Input: part model. Units: mm. Frame: model coordinates. Face numbers are marked on the shaded views. A direction names the side the tool comes from. Coordinates: 2 decimals unless noted, no trailing zeros. Write each loop counter-clockwise with the first axis right and the second up, starting at its lowest first coordinate (ties: lowest second). Pieces come first, ordered by that corner, then holes. Notation, with made-up numbers: M 48.25,-13 L 91.25,-13 A8 cw 91.25,-7 Z; hole C 52,-38 d2. An arc over 180 degrees is marked long. Write each question's results on one line, items separated by ' | '. Start each with the question number.
1. Section query D-D, the plane z = 7.5. Output: boundary loops of the cut face in (x, y).
2. Section query A-A, the plane x = 15.5. Count the separate pieces of the cut face and the enclosed holes in it, and give its area (3 significant figures).
3. Ray query, probe 1 along Z at (x, y) = (-15.5, -6.1); probe 2 along Y at (x, z) = (14.5, 25.5); probe 3 along Z at (x, y) = (-20.5, -26). Return the intervals inside material, ascending.
4. Section query B-B, the plane y = -21. Output: boundary loops of the cut face in (x, z).
5. First-contact query: pin 1 (4 mm diameter, centred on x = -15.5, z = 15.36, fed in from -Y); pin 2 (1 mm diameter, centred on x = 3, y = -34.5, fed in from +Z). Flat tips, straight axial feed; report the tip coordinate or a pass-through.
6. Set-up query: the marked faces 1 and 2. Return all of +Z, -Z, +X, -X, +Y, -Y with unobstructed straight access to the full face (end or side cutting, diameter ignored); none if empty.
7. Pull-direction query (X, two-part tool) for the marked faces 3, 4 and 5; classes: +X half, -X half, draft (parallel to the pull), parting line (faces both ways), or undercut.
```python
from build123d import *

# Parameters (mm, degrees)
SCHIZZO1_R                             = 1.75
SCHIZZO1_R_2                           = 11.05
SCHIZZO1_R_3                           = 2
BASE_FLANGIA1_DEPTH                    = 4
PIEGATURA_START                        = -3.5
PIEGATURA_DELLO_SCHIZZO1_OUTLINE_W     = 50
PIEGATURA_DELLO_SCHIZZO1_OUTLINE_H     = 4
PIEGATURA_DELLO_SCHIZZO1_DEPTH         = 51
PIEGATURA_START_2                      = -7.5
PIEGATURA_DELLO_SCHIZZO1_2_OUTLINE_R   = 1.75
PIEGATURA_DELLO_SCHIZZO1_2_OUTLINE_R_2 = 11.05
PIEGATURA_DELLO_SCHIZZO1_2_DEPTH       = 4
PIEGATURA_START_3                      = -26
PIEGATURA_DELLO_SCHIZZO1_3_DEPTH       = 52
PIEGATURA_START_4                      = -25
PIEGATURA_DELLO_SCHIZZO1_4_DEPTH       = 50
ESTRUSIONE_ESTRUSIONE1_DEPTH           = 2


with BuildPart() as part:
    # Base-Flangia1: sheet metal written as solids
    # Schizzo1 → Base-Flangia1 (new body)
    with BuildSketch(Plane.XY):
        with BuildLine():
            Line((-25, 42.5), (-20, 47.5))
            Line((-20, 47.5), (20, 47.5))
            Line((20, 47.5), (25, 42.5))
            Line((25, 42.5), (25, -42.5))
            ThreePointArc((25, -42.5), (23.535533906, -46.035533906), (20, -47.5))
            Line((20, -47.5), (-20, -47.5))
            ThreePointArc((-20, -47.5), (-23.535533906, -46.035533906), (-25, -42.5))
            Line((-25, -42.5), (-25, 42.5))
        make_face()
        with Locations((-15.5, 42)):
            Circle(SCHIZZO1_R, mode=Mode.SUBTRACT)
        with Locations((15.5, 42)):
            Circle(SCHIZZO1_R, mode=Mode.SUBTRACT)
        with Locations((15.5, 11)):
            Circle(SCHIZZO1_R, mode=Mode.SUBTRACT)
        with Locations((-15.5, 11)):
            Circle(SCHIZZO1_R, mode=Mode.SUBTRACT)
        with Locations((0, 26.5)):
            Circle(SCHIZZO1_R_2, mode=Mode.SUBTRACT)
        with Locations((-12.5, -37.5)):
            Circle(SCHIZZO1_R_3, mode=Mode.SUBTRACT)
        with Locations((12.5, -37.5)):
            Circle(SCHIZZO1_R_3, mode=Mode.SUBTRACT)
    extrude(amount=-BASE_FLANGIA1_DEPTH)

    # Piegatura dello schizzo1: read off the stored shape, not the designer's step
    # Piegatura dello schizzo1 outline → Piegatura dello schizzo1 (cut)
    with BuildSketch(Plane(origin=(0, 0, 0), x_dir=(1, 0, 0), z_dir=(0, 1, 0)).offset(PIEGATURA_START)):
        with Locations((0, 2)):
            Rectangle(PIEGATURA_DELLO_SCHIZZO1_OUTLINE_W, PIEGATURA_DELLO_SCHIZZO1_OUTLINE_H)
    extrude(amount=PIEGATURA_DELLO_SCHIZZO1_DEPTH, mode=Mode.SUBTRACT)

    # Piegatura dello schizzo1 2 outline → Piegatura dello schizzo1 2 (add)
    with BuildSketch(Plane(origin=(0, 0, 0), x_dir=(1, 0, 0), z_dir=(0, 1, 0)).offset(PIEGATURA_START_2)):
        Polygon((-25, 0), (-25, -46.862699383), (-20, -51.862699383), (20, -51.862699383), (25, -46.862699383), (25, 0), align=None)
        with Locations((-15.5, -46.362699383)):
            Circle(PIEGATURA_DELLO_SCHIZZO1_2_OUTLINE_R, mode=Mode.SUBTRACT)
        with Locations((15.5, -46.362699383)):
            Circle(PIEGATURA_DELLO_SCHIZZO1_2_OUTLINE_R, mode=Mode.SUBTRACT)
        with Locations((0, -30.862699383)):
            Circle(PIEGATURA_DELLO_SCHIZZO1_2_OUTLINE_R_2, mode=Mode.SUBTRACT)
        with Locations((-15.5, -15.362699383)):
            Circle(PIEGATURA_DELLO_SCHIZZO1_2_OUTLINE_R, mode=Mode.SUBTRACT)
        with Locations((15.5, -15.362699383)):
            Circle(PIEGATURA_DELLO_SCHIZZO1_2_OUTLINE_R, mode=Mode.SUBTRACT)
    extrude(amount=PIEGATURA_DELLO_SCHIZZO1_2_DEPTH)

    # Piegatura dello schizzo1 3 outline → Piegatura dello schizzo1 3 (cut)
    with BuildSketch(Plane.YZ.offset(PIEGATURA_START_3)):
        with BuildLine():
            ThreePointArc((-3.5, 0.01), (-4.674501807, -2.825498193), (-7.51, -4))
            Line((-7.51, -4), (-3.5, -4))
            Line((-3.5, -4), (-3.5, 0.01))
        make_face()
    extrude(amount=PIEGATURA_DELLO_SCHIZZO1_3_DEPTH, mode=Mode.SUBTRACT)

    # Piegatura dello schizzo1 4 outline → Piegatura dello schizzo1 4 (add)
    with BuildSketch(Plane.YZ.offset(PIEGATURA_START_4)):
        with BuildLine():
            ThreePointArc((-7.5, 0.01), (-7.502928932, 0.002928932), (-7.51, 0))
            Line((-7.51, 0), (-7.5, 0))
            Line((-7.5, 0), (-7.5, 0.01))
        make_face()
    extrude(amount=PIEGATURA_DELLO_SCHIZZO1_4_DEPTH)

    # Schizzo13 → Estrusione-Estrusione1 (add)
    with BuildSketch(Plane.ZY.offset(25)):
        with BuildLine():
            Line((0.01, -7.5), (15, -7.5))
            Line((15, -7.5), (0, -22.5))
            Line((0, -22.5), (0, -7.51))
            ThreePointArc((0, -7.51), (0.002928932, -7.502928932), (0.01, -7.5))
        make_face()
    estrusione_estrusione1 = extrude(amount=-ESTRUSIONE_ESTRUSIONE1_DEPTH)

    # Specchia1: Estrusione-Estrusione1 across plane
    add(estrusione_estrusione1.mirror(Plane(origin=(0, 0, 0), x_dir=(0, 0, 1), z_dir=(1, 0, 0))))


solid = part.part
```
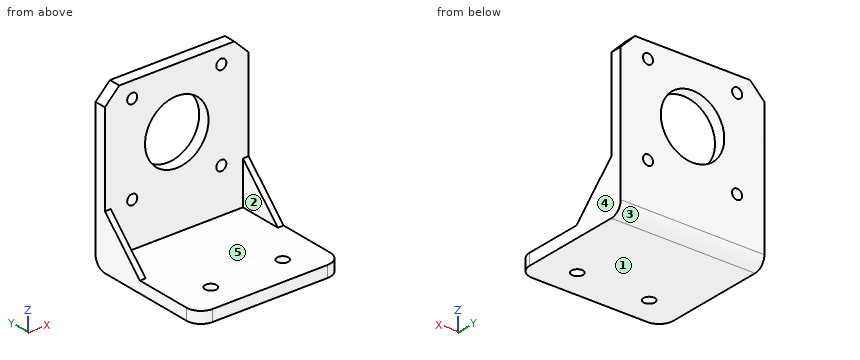
Answer:
1) outline: M -25,-15 L -23,-15 L -23,-7.5 L 23,-7.5 L 23,-15 L 25,-15 L 25,-3.5 L -25,-3.5 Z
2) separate pieces: 3 | enclosed holes: 0 | area: 352 mm^2
3) probe 1: -3.74 to 13.61, 17.11 to 44.61, 48.11 to 51.86 | probe 2: -7.5 to -3.5 | probe 3: -4 to 0
4) outline: M -25,-4 L 25,-4 L 25,1.5 L 23,1.5 L 23,0 L -23,0 L -23,1.5 L -25,1.5 Z
5) pin 1: y = -7.5 | pin 2: z = 0
6) face 1: -Z, +X, -X, +Y, -Y | face 2: +Z, -Y
7) face 3: draft | face 4: +X half | face 5: undercut
